Source: CAD feature listing. Evaluate the final solid. Frame: model axes, mm. A direction names the side the tool comes from. Give positions to 0.01 mm unless a question says otherwise; leave off trailing zeros. Write each loop counter-clockwise with the first axis right and the second up, starting at its lowest first coordinate (ties: lowest second). Pieces come first, ordered by that corner, then holes. Notation, with made-up numbers: (53, 8.25) - (91, 8.25) arc R10 ccw to (91, 20.25) - close; hole circle Ø7 at (35, -1). An arc over 180 degrees is marked (long way). One line per question, with ' | ' between items. Start each with the question number.
(1) Draft query along Y for faces 4 (the flat face through (0, -6, 5)), 5 (the flat face through (0, 3.016, 5)), 6 (the flat face through (0, -3, 10)). Return one class per face: +Y half, -Y half, draft (parallel to the pull), parting line (faces both ways), or undercut.
(2) Section D-D, the plane x = 6.75. Return loops of the section in (y, z), plus the area to 3 significant figures.
(3) Section A-A, the plane x = 2.5. Return loops of the section in (y, z).
(4) Section B-B, the plane z = 3. Return loops of the section in (x, y), plus the area to 3 significant figures.
(5) Pin query (flat end, axial travel): pin 1 (6 mm diameter, centred on x = -3.5, y = -0.5, fed in from -Z); pin 2 (5 mm diameter, centred on y = 3.5, z = 6, fed in from -X); pin 3 (3 mm diameter, centred on x = 3, y = 0, fed in from +Z); pin 4 (1.1 mm diameter, centred on y = 2, z = 0.5, fed in from +X). Return the tip coordinate at first contact, or that it passes through.
(6) Section C-C, the plane y = 1.25. Return loops of the section in (x, z).
(7) Ray query, line 1 (Y direction, x = -1.75, z = 8.75); line 2 (X direction, y = 0, z = 5.75); line 3 (Y direction, x = -2.25, z = 0.5). Return the intervals inside material, ascending. Write a range as [from, to].
(8) Access query for faces 1 (the flat face through (-5.1, 0.516, 0.5)), 2 (the cylindrical face through (-9.35, -0.09, 5.07)), 3 (the flat face through (0, -2.484, 5)). Directions: +Z, -Z, +X, -X, +Y, -Y. A direction counts if a zero-diameter tool reaches every point of the face in a straight line with its end or side. Return the directions, or none.
```python
from build123d import *

# Parameters (mm, degrees)
F0_W     = 22
F0_H     = 12
F1_DEPTH = 1
F2_DEPTH = 10
F3_W     = 2.4
F3_H     = 2.5
F4_DEPTH = 9
F5_R     = 2
F6_R     = 12.5
F7_DEPTH = 25
F8_W     = 3.05
F8_H     = 1
F9_DEPTH = 25


with BuildPart() as f1:
    # F0 (on Top) → F1 (new body)
    with BuildSketch(Plane.XY):
        Rectangle(F0_W, F0_H)
        Polygon((-5.85, 3.0159242167), (0, 3.0159242167), (5.85, 3.0159242167), (5.85, 0.5159242167), (8.6, 0.5159242167), (8.6, -2.4840757833), (0, -2.4840757833), (-8.6, -2.4840757833), (-8.6, 0.5159242167), (-5.85, 0.5159242167), align=None, mode=Mode.SUBTRACT)
        Polygon((8.6, 0.5159242167), (5.85, 0.5159242167), (-5.85, 0.5159242167), (-8.6, 0.5159242167), (-8.6, -2.4840757833), (0, -2.4840757833), (8.6, -2.4840757833), align=None)
    extrude(amount=F1_DEPTH)

    # F0 (on Top) → F2 (join)
    with BuildSketch(Plane.XY):
        Rectangle(F0_W, F0_H)
        Polygon((-5.85, 3.0159242167), (0, 3.0159242167), (5.85, 3.0159242167), (5.85, 0.5159242167), (8.6, 0.5159242167), (8.6, -2.4840757833), (0, -2.4840757833), (-8.6, -2.4840757833), (-8.6, 0.5159242167), (-5.85, 0.5159242167), align=None, mode=Mode.SUBTRACT)
    extrude(amount=F2_DEPTH)

    # F3 (on face) → F4 (cut, through all)
    with BuildSketch(Plane.XY.offset(10)):
        with Locations((-7.05, 1.7659242167)):
            Rectangle(F3_W, F3_H)
        with Locations((7.05, 1.7659242167)):
            Rectangle(F3_W, F3_H)
    extrude(amount=-F4_DEPTH, mode=Mode.SUBTRACT)

    # F5
    f5_edges = [f1.edges().sort_by_distance(p)[0] for p in [
        (-11, -6, 5),
        (11, -6, 5),
        (-11, 6, 5),
        (11, 6, 5),
    ]]
    fillet(f5_edges, radius=F5_R)

    # F6 (on face) → F7 (cut)
    with BuildSketch(Plane.XY.offset(10)):
        Circle(F6_R)
        with BuildLine():
            ThreePointArc((-7.1709483334, 6), (0, 9.35), (7.1709483334, 6))
            Line((7.1709483334, 6), (9, 6))
            ThreePointArc((9, 6), (10.4142135624, 5.4142135624), (11, 4))
            Line((11, 4), (11, -4))
            ThreePointArc((11, -4), (10.4142135624, -5.4142135624), (9, -6))
            Line((9, -6), (7.1709483334, -6))
            ThreePointArc((7.1709483334, -6), (0, -9.35), (-7.1709483334, -6))
            Line((-7.1709483334, -6), (-9, -6))
            ThreePointArc((-9, -6), (-10.4142135624, -5.4142135624), (-11, -4))
            Line((-11, -4), (-11, 4))
            ThreePointArc((-11, 4), (-10.4142135624, 5.4142135624), (-9, 6))
            Line((-9, 6), (-7.1709483334, 6))
        make_face(mode=Mode.SUBTRACT)
        with BuildLine():
            ThreePointArc((-7.1709483334, -6), (-9.35, 0), (-7.1709483334, 6))
            Line((-7.1709483334, 6), (-9, 6))
            ThreePointArc((-9, 6), (-10.4142135624, 5.4142135624), (-11, 4))
            Line((-11, 4), (-11, -4))
            ThreePointArc((-11, -4), (-10.4142135624, -5.4142135624), (-9, -6))
            Line((-9, -6), (-7.1709483334, -6))
        make_face()
        with BuildLine():
            ThreePointArc((7.1709483334, 6), (8.788369215, 3.1917184308), (9.35, 0))
            ThreePointArc((9.35, 0), (8.788369215, -3.1917184308), (7.1709483334, -6))
            Line((7.1709483334, -6), (9, -6))
            ThreePointArc((9, -6), (10.4142135624, -5.4142135624), (11, -4))
            Line((11, -4), (11, 4))
            ThreePointArc((11, 4), (10.4142135624, 5.4142135624), (9, 6))
            Line((9, 6), (7.1709483334, 6))
        make_face()
    extrude(amount=-F7_DEPTH, mode=Mode.SUBTRACT)

    # F8 (on face) → F9 (cut)
    with BuildSketch(Plane.XY.offset(1)):
        with Locations((-2.825, 0.0159242167)):
            Rectangle(F8_W, F8_H)
        with Locations((2.825, 0.0159242167)):
            Rectangle(F8_W, F8_H)
    extrude(amount=-F9_DEPTH, mode=Mode.SUBTRACT)


solid = f1.part
```
Check sheet entries:
1) face 4: -Y half | face 5: undercut | face 6: draft
2) outline: (-6, 0) - (6, 0) - (6, 10) - (3.02, 10) - (3.02, 1) - (-2.48, 1) - (-2.48, 10) - (-6, 10) - close | area: 70.5 mm²
3) outline: (-6, 0) - (-0.48, 0) - (-0.48, 1) - (-2.48, 1) - (-2.48, 10) - (-6, 10) - close; (3.02, 0) - (6, 0) - (6, 10) - (3.02, 10) - close
4) outline: (-7.17, -6) - (7.17, -6) arc R9.35 ccw to (7.17, 6) - (-7.17, 6) arc R9.35 ccw to start; hole (-8.6, -2.48) - (8.6, -2.48) - (8.6, 0.52) - (8.25, 0.52) - (8.25, 3.02) - (-8.25, 3.02) - (-8.25, 0.52) - (-8.6, 0.52) - close | area: 115 mm²
5) pin 1: z = 0 | pin 2: x = -9.3 | pin 3: z = 1 | pin 4: x = 9.24
6) outline: (-9.27, 0) - (-5.85, 0) - (-5.85, 1) - (-8.25, 1) - (-8.25, 10) - (-9.27, 10) - close; (5.85, 0) - (9.27, 0) - (9.27, 10) - (8.25, 10) - (8.25, 1) - (5.85, 1) - close
7) line 1: [-6, -2.48], [3.02, 6] | line 2: [-9.35, -8.6], [8.6, 9.35] | line 3: [-6, -0.48], [3.02, 6]
8) face 1: +Z, -Z | face 2: +Z, -Z, -X | face 3: +Z
